Can you work these out from the model? Positions are in its coordinate system, mm. Coordinates: 2 decimals unless noted, no trailing zeros. Loops run counter-clockwise (first coordinate to the right, second up) from the corner with the lowest first, then second, coordinate; pieces in that order, holes last.
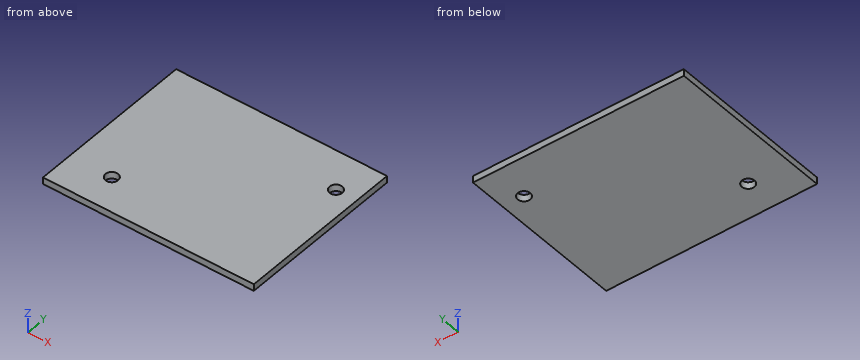
Autodesk Inventor part; units mm, degrees
ref_plane "YZ Plane" through (0, 0, 0) normal (1, 0, 0) x (0, 1, 0)
ref_plane "XZ Plane" through (0, 0, 0) normal (0, 1, 0) x (-1, 0, 0)
ref_plane "XY Plane" through (0, 0, 0) normal (0, 0, 1) x (1, 0, 0)
sketch "Sketch1" plane through (0, 0, 0) normal (0, 0, 1) x (1, 0, 0)
  line L0 (25, -20) -> (-25, -20)
  line L1 (-25, -20) -> (-25, 20)
  line L2 (-25, 20) -> (25, 20)
  line L3 (25, 20) -> (25, -20)
  line L4 (25, 0) -> (-25, 0) construction
  point P0 (0, 0)
  point P1 (0, 0)
  dimension "d0" = 50
  dimension "d1" = 40
extrude "Extrusion1" add sketch "Sketch1" along normal blind 1.6
sketch "Sketch2" plane through (0, 0, 1.6) normal (0, 0, 1) x (1, 0, 0)
  line L0 (-25, 18.8203) -> (25.4554, 18.8203) construction
  line L1 (25.4554, 18.8203) -> (25.4554, -19.9538) construction
  line L2 (25.4554, -19.9538) -> (-25, -19.9538) construction
  line L3 (-25, -19.9538) -> (-25, 18.8203) construction
  point P0 (0, 0)
sketch "Sketch3" plane through (0, 0, 1.6) normal (0, 0, 1) x (1, 0, 0)
  line L0 (-25, -20) -> (-25, 20)
  line L1 (25, -20) -> (-25, -20)
  point P0 (0, 0)
  point P1 (-15, -12)
  point P2 (20, 11)
  dimension "d5" = 8
  dimension "d6" = 10
  dimension "d7" = 45
  dimension "d8" = 31
hole "Hole1" at (20, 11, 1.6) at (-15, -12, 1.6) direction (0, 0, -1) diameter 3 end through all
properties part number "BOARD_IMAGE"
Item 1: I need wall thicknesses on line 1 along X through (y, z) = (-12, 1.05); line 2 along X through (y, z) = (11, 1.15); line 3 along Y through (x, z) = (-15, 0.5). Which ranges of each line are inside material? Lowest first, please.
Results are:
line 1: x = -25 to -16.5, -13.5 to 25
line 2: x = -25 to 18.5, 21.5 to 25
line 3: y = -20 to -13.5, -10.5 to 20
Item 2: I'm going to push a flat-ended pin straight in: P1, Ø5, axis at x = -15, y = -12, coming from the +Z side. Where does the tip first touch, or does it pass through?
Results are:
P1: stops at z = 1.6
Item 3: Suppose I cut it at A-A, the plane x = -15. Please give me the cut outline in (y, z).
Results are:
outline: (-20, 0) - (-13.5, 0) - (-13.5, 1.6) - (-20, 1.6) - close; (-10.5, 0) - (20, 0) - (20, 1.6) - (-10.5, 1.6) - close
Item 4: Suppose I cut it at B-B, the plane y = 11. Please give me the cut outline in (x, z).
Results are:
outline: (-25, 0) - (18.5, 0) - (18.5, 1.6) - (-25, 1.6) - close; (21.5, 0) - (25, 0) - (25, 1.6) - (21.5, 1.6) - close
